Read the model definition and answer for the solid it produces. Units are mm, in the model's axes. Face numbers are marked on the shaded views. A direction names the side the tool comes from. Round coordinates to 2 decimals unless told otherwise and drop trailing zeros. Order: outer loops, then holes, each group sorted by start corner. A loop starts at its lowest first (then second) coordinate and runs counter-clockwise, first axis right, second up. Notation, with made-up numbers: (31.25, -29.5) -> (66.25, -29.5) arc R29 cw to (66.25, 9.5) -> close; hole circle Ø1 at (73, 13). An arc over 180 degrees is marked (long way). Answer as a JSON object with one key per item and string values. Group by question number.
Item 1: Section A-A, the plane x = 0 is taken. Write down the section's boundary in (y, z), plus the area to 4 significant figures.
Item 2: For the marked faces 1 and 2, determine the directions among +Z, -Z, +X, -X, +Y, -Y from which every point of the face is accessible in a straight line to the end or side of a thin tool.
Item 3: Section C-C, the plane z = 2.55 is taken. Write down the section's boundary in (x, y).
Item 4: Consider probe 1 along Z at (x, y) = (-1, -4.5); probe 2 along Y at (x, z) = (2, 1.3); probe 3 along X at (y, z) = (1.5, 3.5). Determine where each line is inside the solid, lowest interval first. Write a range as from..to.
Item 5: Section D-D, the plane y = -3.25 is taken. Write down the section's boundary in (x, z), plus the area to 3 significant figures.
Item 6: Section B-B, the plane y = 0 is taken. Write down the section's boundary in (x, z), plus the area to 4 significant figures.
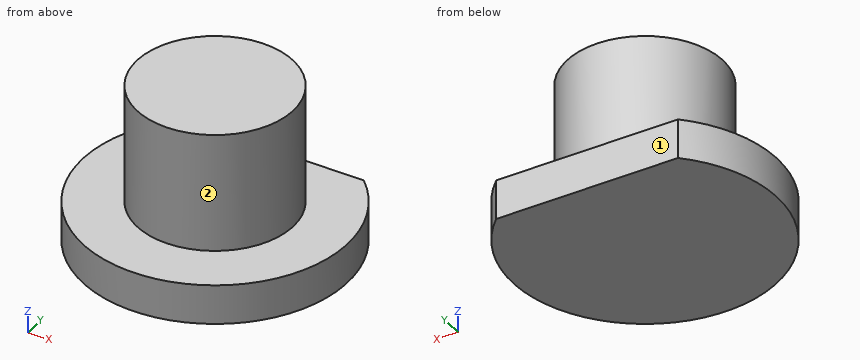
from build123d import *

# Parameters (mm, degrees)
SKETCH1_R           = 2.95
BOSS_EXTRUDE1_DEPTH = 4.5
SKETCH1_5_R         = 2.95
BOSS_EXTRUDE2_DEPTH = 1.5
BOSS_EXTRUDE3_START = 1.5
SKETCH3_R           = 2.95
BOSS_EXTRUDE3_DEPTH = 1.5


with BuildPart() as part:
    # Sketch1 → Boss-Extrude1 (new body)
    with BuildSketch(Plane.XY):
        Circle(SKETCH1_R)
    extrude(amount=BOSS_EXTRUDE1_DEPTH)



with BuildPart() as body_2:
    # Sketch1_5 → Boss-Extrude2 (new body)
    with BuildSketch(Plane.XY):
        with BuildLine():
            Line((-3.469870315, 3.6), (3.469870315, 3.6))
            ThreePointArc((3.469870315, 3.6), (0, -5), (-3.469870315, 3.6))
        make_face()
        Circle(SKETCH1_5_R, mode=Mode.SUBTRACT)
    extrude(amount=-BOSS_EXTRUDE2_DEPTH)


with BuildPart() as part_1:
    add(part.part)

    add(body_2.part)  # Boss-Extrude3 merges body 2
    # Sketch3 → Boss-Extrude3 (add)
    with BuildSketch(Plane(origin=(0, 0, 0), x_dir=(-1, 0, 0), z_dir=(0, 0, -1)).offset(BOSS_EXTRUDE3_START)):
        with Locations(Location((0, 0, 0), (0, 0, 180))):
            Circle(SKETCH3_R)
    extrude(amount=-BOSS_EXTRUDE3_DEPTH)


solid = part_1.part
Values found:
{
 "1": {"outline": "(-5, -1.5) -> (3.6, -1.5) -> (3.6, 0) -> (2.95, 0) -> (2.95, 4.5) -> (-2.95, 4.5) -> (-2.95, 0) -> (-5, 0) -> close", "area": "39.45 mm2"},
 "2": {"face 1": "+Z, -Z, +X, -X, +Y", "face 2": "+Z"},
 "3": {"outline": "circle Ø5.9 at (0, 0)"},
 "4": {"probe 1": "-1.5..0", "probe 2": "-2.17..2.17", "probe 3": "-2.54..2.54"},
 "5": {"outline": "(-3.8, -1.5) -> (3.8, -1.5) -> (3.8, 0) -> (-3.8, 0) -> close", "area": "11.4 mm2"},
 "6": {"outline": "(-5, -1.5) -> (5, -1.5) -> (5, 0) -> (2.95, 0) -> (2.95, 4.5) -> (-2.95, 4.5) -> (-2.95, 0) -> (-5, 0) -> close", "area": "41.55 mm2"}
}
